Read the model definition and answer for the solid it produces. Units are mm, in the model's axes. A direction names the side the tool comes from. Give positions to 0.01 mm unless a question says otherwise; leave off trailing zeros. Loops run counter-clockwise (first coordinate to the right, second up) from the corner with the lowest first, then second, coordinate; pieces in that order, holes last. Notation, with made-up numbers: (-24, 67.25) - (25, 67.25) arc R22 ccw to (25, 77.25) - close; hole circle Ø8 at (-13.5, 77). An arc over 180 degrees is marked (long way). Write item = value, one per line. Start each with the question number.
from build123d import *

# Parameters (mm, degrees)
TORUS_R               = 2
TORUS_ANGLE           = 120
TORUS_PLACEMENT_ANGLE = 209
CYLINDER002_R         = 4
CYLINDER002_DEPTH     = 10
CYLINDER001_R         = 4
CYLINDER001_DEPTH     = 10
CYLINDER_R            = 50
CYLINDER_DEPTH        = 3


with BuildPart() as torus:
    # Torus → Torus (revolve)
    with BuildSketch(Plane.XZ):
        with Locations((22, 0)):
            Circle(TORUS_R)
    revolve(axis=Axis((0, 0, 0), (0, 0, 1)), revolution_arc=TORUS_ANGLE)


with BuildPart() as torus_1:
    # Torus placement: moved
    add(torus.part.moved(Location((0, 0, 2))).rotate(Axis((0, 0, 2), (0, 0, 1)), TORUS_PLACEMENT_ANGLE))


with BuildPart() as cylinder001:
    # Cylinder002 → Cylinder002 (new body)
    with BuildSketch(Plane(origin=(18, 22, 1), x_dir=(1, 0, 0), z_dir=(0, 0, 1))):
        Circle(CYLINDER002_R)
    extrude(amount=CYLINDER002_DEPTH)


with BuildPart() as ojos_boca:
    # Cylinder001 → Cylinder001 (new body)
    with BuildSketch(Plane(origin=(-20, 22, 1), x_dir=(1, 0, 0), z_dir=(0, 0, 1))):
        Circle(CYLINDER001_R)
    extrude(amount=CYLINDER001_DEPTH)

    # Fusion: union Cylinder001
    add(cylinder001.part)

    # Fusion001: union Torus
    add(torus_1.part)


with BuildPart() as smiley:
    # Cylinder → Cylinder (new body)
    with BuildSketch(Plane.XY):
        Circle(CYLINDER_R)
    extrude(amount=CYLINDER_DEPTH)

    # Cut: cut Ojos_Boca
    add(ojos_boca.part, mode=Mode.SUBTRACT)


solid = smiley.part
1. Given P1, Ø6.5, axis at x = 17.5, y = 21.5, coming from the +Z side, flat-ended and moving along its own axis, determine where the tip first touches the part or whether it passes through.
2. A cutting plane is placed at A-A on z = 2. Give the vertices of the cut face in (x, y), and give its area (3 significant figures).
3. For a pull along X with two mould halves and no side action, classify faces 1 (the cylindrical face through (47.69, 15.02, 1.48)), 2 (the flat face through (-1, 1, 0)), 3 (the cylindrical face through (17.479, 25.966, 1.986)), 4 (the cylindrical face through (-20.521, 25.966, 1.986)) as released by +X, released by -X, zero draft, split by the parting line, or undercut.
4. A cutting plane is placed at C-C on y = 22. Give the vertices of the cut face in (x, z), and give its area (3 significant figures).
5. Consider line 1 along Y through (x, z) = (-20, 1.9); line 2 along Y through (x, z) = (18, 2.4); line 3 along X through (y, z) = (19, 1.9). Determine where each line is inside the solid, lowest interval first. Write a range as [from, to].
6. A tool of negligible diameter and unlimited length cuts with its end or side. For faces 5 (the flat face through (-19.217, -10.652, 1.854)), 6 (the flat face through (-1, 1, 3)), 7 (the flat face through (18, 22, 1)), from which of +Z, -Z, +X, -X, +Y, -Y can it reach the whole face along a straight path? Write none if from no direction.
Reply:
q1.P1 = 1
q2.outline = circle Ø100 at (0, 0); hole circle Ø8 at (-20, 22); hole (-20.99, -11.64) arc R24 ccw to (20.57, -12.36) - (17.14, -10.3) arc R20 cw to (-17.49, -9.7) - close; hole circle Ø8 at (18, 22)
q2.area = 7,570 mm^2
q3.face_1 = split by the parting line
q3.face_2 = zero draft
q3.face_3 = undercut
q3.face_4 = undercut
q4.outline = (-44.9, 0) - (44.9, 0) - (44.9, 3) - (22, 3) - (22, 1) - (14, 1) - (14, 3) - (-16, 3) - (-16, 1) - (-24, 1) - (-24, 3) - (-44.9, 3) - close
q4.area = 237 mm^2
q5.line_1 = [-45.83, -13.26], [-11.09, 18], [26, 45.83]
q5.line_2 = [-46.65, -15.81], [-10.82, 18], [26, 46.65]
q5.line_3 = [-46.25, -22.65], [-17.35, 15.35], [20.65, 46.25]
q6.face_5 = none
q6.face_6 = +Z, +X, -X, +Y, -Y
q6.face_7 = +Z
